from build123d import *

# Parameters (mm, degrees)
F1_DEPTH = 6.35
F2_R     = 2.54


with BuildPart() as f1:
    # F0 (on Front) → F1 (new body, symmetric)
    with BuildSketch(Plane.XZ):
        Polygon((-8.977415, 45.314699), (-15.062025, 45.314699), (-15.062025, -37.343994), (-9.223152, -37.343994), (-9.223152, 31.330701), (27.435317, -36.294828), (37.48342, -36.294828), (37.48342, 48.394047), (31.835622, 48.394047), (31.835622, -29.974949), align=None)
    extrude(amount=F1_DEPTH, both=True)

    # F2
    f2_edges = [f1.edges().sort_by_distance(p)[0] for p in [
        (-15.062025, 0, -37.343994),
        (37.48342, 0, 48.394047),
        (-15.062025, 0, 45.314699),
        (31.835622, 0, 48.394047),
        (-9.223152, 0, -37.343994),
        (37.48342, 0, -36.294828),
        (27.435317, 0, -36.294828),
        (-8.977415, 0, 45.314699),
    ]]
    fillet(f2_edges, radius=F2_R)


solid = f1.part
The listing builds one solid part. Answer for the finished solid, in the listing's coordinates (mm). A direction names the side the tool comes from. Give positions to 0.01 mm unless a question says otherwise; leave off trailing zeros. Loops run counter-clockwise (first coordinate to the right, second up) from the corner with the lowest first, then second, coordinate; pieces in that order, holes last.
Item 1: A tool of negligible diameter and unlimited length cuts with its end or side. For faces 5 (the cylindrical face through (-9.95, -0.09, -36.58)), 6 (the flat face through (32, 0, -36.295)), 7 (the flat face through (-11, 0, 45.315)), from which of +Z, -Z, +X, -X, +Y, -Y can it reach the whole face along a straight path? Write none if from no direction.
Derived:
face 5: -Z, +Y, -Y
face 6: -Z, +X, +Y, -Y
face 7: +Z, -X, +Y, -Y
Item 2: A cutting plane is placed at D-D (x = 30). Give the vertices of the cut face in (y, z), then the cut area to 3 significant figures.
Derived:
outline: (-6.35, -36.29) - (6.35, -36.29) - (6.35, -26.59) - (-6.35, -26.59) - close
area: 123 mm2
Item 3: Find the intervals of material crossed by line 1 along X through (y, z) = (2.75, -1.5); line 2 along X through (y, z) = (-2.5, -24); line 3 along X through (y, z) = (-4, 31.5), in increasing order.
Derived:
line 1: x = -15.06 to -9.22, 8.57 to 16.4, 31.84 to 37.48
line 2: x = -15.06 to -9.22, 20.77 to 28.6, 31.84 to 37.48
line 3: x = -15.06 to -1.49, 31.84 to 37.48
Item 4: A cutting plane is placed at C-C (z = 36). Give the vertices of the cut face in (x, y), then the cut area to 3 significant figures.
Derived:
outline: (-15.06, -6.35) - (-3.93, -6.35) - (-3.93, 6.35) - (-15.06, 6.35) - close; (31.84, -6.35) - (37.48, -6.35) - (37.48, 6.35) - (31.84, 6.35) - close
area: 213 mm2
Item 5: A cutting plane is placed at A-A (z = -20). Give the vertices of the cut face in (x, y), then the cut area to 3 significant figures.
Derived:
outline: (-15.06, -6.35) - (-9.22, -6.35) - (-9.22, 6.35) - (-15.06, 6.35) - close; (18.6, -6.35) - (26.43, -6.35) - (26.43, 6.35) - (18.6, 6.35) - close; (31.84, -6.35) - (37.48, -6.35) - (37.48, 6.35) - (31.84, 6.35) - close
area: 245 mm2
Item 6: Each of these flat-tipped pins is pushed along its axis until it touches: pin 1 Ø1 at (x, y) = (-0.5, -3.5) entering from -Z; pin 2 Ø6.5 at (x, y) = (33, 3) entering from -Z; pin 3 Ø4 at (x, y) = (12.5, -3) entering from +Z; pin 4 Ø12 at (x, z) = (8, -24.5) entering from -Y. Where does it stop, or does it pass through?
Derived:
pin 1: stops at z = 14.32
pin 2: stops at z = -36.29
pin 3: stops at z = 9.38
pin 4: passes through
Item 7: Determine the mould class of faces 1 (the flat face through (8.494, -0.089, -1.353)), 2 (the cylindrical face through (27.665, -0.089, -35.947)), 3 (the flat face through (11, 6.35, 6)), 4 (the cylindrical face through (-14.3, -0.09, 44.59)) for opening direction X: +X half, -X half, draft (parallel to the pull), parting line (faces both ways), or undercut.
Derived:
face 1: undercut
face 2: undercut
face 3: draft
face 4: -X half
Item 8: A cutting plane is placed at B-B (y = 5.25). Give the vertices of the cut face in (x, z), then the cut area to 3 significant figures.
Derived:
outline: (-15.06, -34.8) arc R2.54 ccw to (-12.52, -37.34) - (-11.76, -37.34) arc R2.54 ccw to (-9.22, -34.8) - (-9.22, 31.33) - (26.71, -34.97) arc R2.54 ccw to (28.95, -36.29) - (34.94, -36.29) arc R2.54 ccw to (37.48, -33.75) - (37.48, 45.85) arc R2.54 ccw to (34.94, 48.39) - (34.38, 48.39) arc R2.54 ccw to (31.84, 45.85) - (31.84, -29.97) - (-8.26, 43.99) arc R2.54 ccw to (-10.49, 45.31) - (-12.52, 45.31) arc R2.54 ccw to (-15.06, 42.77) - close
area: 1,530 mm2
